Autodesk Inventor part; units mm, degrees
ref_plane "YZ Plane" through (0, 0, 0) normal (1, 0, 0) x (0, 1, 0)
ref_plane "XZ Plane" through (0, 0, 0) normal (0, 1, 0) x (-1, 0, 0)
ref_plane "XY Plane" through (0, 0, 0) normal (0, 0, 1) x (1, 0, 0)
sketch "Boceto1" plane through (0, 0, 0) normal (0, 0, 1) x (1, 0, 0)
  line L0 (0, 0) -> (19.9, 0)
  line L1 (19.9, 0) -> (19.9, 22.1)
  line L2 (19.9, 22.1) -> (0, 22.1)
  line L3 (0, 22.1) -> (0, 0)
  circle A0 centre (9.95, 11.05) radius 8.2
  dimension "d0" = 19.9
  dimension "d1" = 22.1
  dimension "d2" = 16.4
extrude "Extrusión1" add sketch "Boceto1" along normal blind 1
extrude "Extrusión2" add sketch "Boceto1" along normal blind 15.5 contours A0
fillet "Empalme1" radius 1 1 edges at (1.75, 11.05, 15.5)
properties part number "LV-MaxSonar-EZ"
Verification items for the finished model (mm, model axes). A direction names the side the tool comes from. Round coordinates to 2 decimals unless told otherwise and drop trailing zeros. Loops run counter-clockwise (first coordinate to the right, second up) from the corner with the lowest first, then second, coordinate; pieces in that order, holes last. Notation, with made-up numbers: (48.25, -37) - (58.25, -37) arc R30 cw to (58.25, -6) - close; hole circle Ø7 at (83.25, 20). An arc over 180 degrees is marked (long way). Write item = value, one per line.
Q1. Sectioned sample at B-B on y = 11.05. Record the boundary of the cut face in (x, z).
Here are the results:
outline = (0, 0) - (19.9, 0) - (19.9, 1) - (18.15, 1) - (18.15, 14.5) arc R1 ccw to (17.15, 15.5) - (2.75, 15.5) arc R1 ccw to (1.75, 14.5) - (1.75, 1) - (0, 1) - close
Q2. Material ranges on L1, parallel to Z at x = 16.5, y = 1.5; L2, parallel to X at y = 10.75, z = 10; L3, parallel to Y at x = 16.25, z = 6.25, recorded low to high.
Here are the results:
L1 = 0 to 1
L2 = 1.76 to 18.14
L3 = 5.8 to 16.3
Q3. Sectioned sample at D-D on x = 18.5. Record the boundary of the cut face in (y, z), plus the area to 3 significant figures.
Here are the results:
outline = (0, 0) - (22.1, 0) - (22.1, 1) - (0, 1) - close
area = 22.1 mm^2
Q4. Tool access check on faces 1 (the flat face through (10.1, 22.1, 0.5)), 2 (the flat face through (3, 16, 1)). Record the directions out of +Z, -Z, +X, -X, +Y, -Y that give a thin tool (end or side, any length) a straight path to the whole face; none if there is none.
Here are the results:
face_1 = +Z, -Z, +X, -X, +Y
face_2 = +Z
Q5. Sectioned sample at C-C on z = 8.5. Record the boundary of the cut face in (x, y).
Here are the results:
outline = circle Ø16.4 at (9.95, 11.05)
Q6. Sectioned sample at A-A on x = 9.95. Record the boundary of the cut face in (y, z).
Here are the results:
outline = (0, 0) - (22.1, 0) - (22.1, 1) - (19.25, 1) - (19.25, 14.5) arc R1 ccw to (18.25, 15.5) - (3.85, 15.5) arc R1 ccw to (2.85, 14.5) - (2.85, 1) - (0, 1) - close
Q7. Depth check by flat-ended pin: pin 1 (3 mm diameter, centred on x = 16, z = 9, fed in from -Y); pin 2 (8 mm diameter, centred on y = 6.5, z = 12.5, fed in from -X); pin 3 (3 mm diameter, centred on x = 16.5, y = 9.5, fed in from -Z); pin 4 (1 mm diameter, centred on y = 7.5, z = 10, fed in from -X). Enter the tip coordinate at first touch or a pass-through.
Here are the results:
pin_1 = 4.23
pin_2 = 1.77
pin_3 = 0
pin_4 = 2.34
